Geometry check sheet. Reference: the model listing, model coordinates, mm. A direction names the side the tool comes from. Round coordinates to 2 decimals unless told otherwise and drop trailing zeros. Write each loop counter-clockwise with the first axis right and the second up, starting at its lowest first coordinate (ties: lowest second). Pieces come first, ordered by that corner, then holes. Notation, with made-up numbers: (6, 5.5) -> (15, 5.5) arc R12 cw to (15, 12.5) -> close; hole circle Ø11 at (83.25, -35). An arc over 180 degrees is marked (long way). Use a Markdown table: item, result.
```python
from build123d import *

# Parameters (mm, degrees)
SKETCH1_R           = 1.5
BOSS_EXTRUDE1_DEPTH = 5
FILLET1_R           = 10
CUT_EXTRUDE1_DEPTH  = 1
CUT_EXTRUDE2_DEPTH  = 3.9


with BuildPart() as part:
    # Sketch1 → Boss-Extrude1 (new, symmetric)
    with BuildSketch(Plane.XY):
        with BuildLine():
            Line((4, 60), (4, -60))
            ThreePointArc((4, -60), (0, -64), (-4, -60))
            ThreePointArc((-4, -60), (-12.339895115, 0), (-4, 60))
            ThreePointArc((-4, 60), (0, 64), (4, 60))
        make_face()
        with Locations((0, 60)):
            Circle(SKETCH1_R, mode=Mode.SUBTRACT)
        with Locations((0, 30)):
            Circle(SKETCH1_R, mode=Mode.SUBTRACT)
        with Locations((0, -30)):
            Circle(SKETCH1_R, mode=Mode.SUBTRACT)
        Circle(SKETCH1_R, mode=Mode.SUBTRACT)
        with Locations((0, -60)):
            Circle(SKETCH1_R, mode=Mode.SUBTRACT)
    extrude(amount=BOSS_EXTRUDE1_DEPTH, both=True)

    # Fillet1
    fillet1_edges = [part.edges().sort_by_distance(p)[0] for p in [
        (-4, -60, 0),
        (-4, 60, 0),
    ]]
    fillet(fillet1_edges, radius=FILLET1_R)

    # Sketch2 → Cut-Extrude1 (cut)
    with BuildSketch(Plane.XY.offset(5)):
        with BuildLine():
            ThreePointArc((-3.293906421, -58.816707776), (-0.342834029, -56.516831209), (3, -58.197224362))
            Line((3, -58.197224362), (3, -31.802775638))
            ThreePointArc((3, -31.802775638), (-3.5, -30), (3, -28.197224362))
            Line((3, -28.197224362), (3, -1.802775638))
            ThreePointArc((3, -1.802775638), (-3.5, 0), (3, 1.802775638))
            Line((3, 1.802775638), (3, 28.197224362))
            ThreePointArc((3, 28.197224362), (-3.5, 30), (3, 31.802775638))
            Line((3, 31.802775638), (3, 58.197224362))
            ThreePointArc((3, 58.197224362), (-0.342834029, 56.516831209), (-3.293906421, 58.816707776))
            ThreePointArc((-3.293906421, 58.816707776), (-11.339895115, 0), (-3.293906421, -58.816707776))
        make_face()
    extrude(amount=-CUT_EXTRUDE1_DEPTH, mode=Mode.SUBTRACT)

    # Sketch3 → Cut-Extrude2 (cut, symmetric)
    with BuildSketch(Plane.XY):
        with BuildLine():
            ThreePointArc((-3.293906421, 58.816707776), (-1.64732722, 64.431350021), (0.148659418, 70))
            Line((0.148659418, 70), (-49.851340582, 70))
            Line((-49.851340582, 70), (-49.851340582, -70))
            Line((-49.851340582, -70), (0.148659418, -70))
            ThreePointArc((0.148659418, -70), (-1.64732722, -64.431350021), (-3.293906421, -58.816707776))
            ThreePointArc((-3.293906421, -58.816707776), (-11.339895115, 0), (-3.293906421, 58.816707776))
        make_face()
    extrude(amount=CUT_EXTRUDE2_DEPTH, both=True, mode=Mode.SUBTRACT)


solid = part.part
```
(1) Thickness scan on line 1 (Y direction, x = 0, z = 0.75); line 2 (Y direction, x = -1, z = 0.75); line 3 (Z direction, x = -6.25, y = -48). Record the ranges inside material, lowest first.
A:
| item | result |
|---|---|
| line 1 | y = -64 to -61.5, -58.5 to -31.5, -28.5 to -1.5, 1.5 to 28.5, 31.5 to 58.5, 61.5 to 64 |
| line 2 | y = -63.87 to -61.12, -58.88 to -31.12, -28.88 to -1.12, 1.12 to 28.88, 31.12 to 58.88, 61.12 to 63.87 |
| line 3 | z = -5 to -3.9, 3.9 to 5 |
(2) Section check D-D on y = -11. Record the cut outline in (x, z).
A:
| item | result |
|---|---|
| outline | (-12.06, -5) -> (4, -5) -> (4, 5) -> (3, 5) -> (3, 4) -> (-11.06, 4) -> (-11.06, 5) -> (-12.06, 5) -> (-12.06, 3.9) -> (-11.06, 3.9) -> (-11.06, -3.9) -> (-12.06, -3.9) -> close |
(3) Release check for a two-part mould opening along Y. For faces 1 (the face through (-12.34, -0.84, 4.46)), 2 (the face through (-0.195, -28.513, -0.07)), 3 (the face through (-12, 0, 3.9)) record: +Y half, -Y half, draft (parallel to the pull), parting line (faces both ways), or undercut.
A:
| item | result |
|---|---|
| face 1 | parting line |
| face 2 | undercut |
| face 3 | draft |
(4) Section check C-C on y = 30. Record the cut outline in (x, z), plus the area to 3 significant figures.
A:
| item | result |
|---|---|
| outline | (-10.28, -5) -> (-1.5, -5) -> (-1.5, 5) -> (-3.5, 5) -> (-3.5, 4) -> (-9.28, 4) -> (-9.28, 5) -> (-10.28, 5) -> (-10.28, 3.9) -> (-9.28, 3.9) -> (-9.28, -3.9) -> (-10.28, -3.9) -> close; (1.5, -5) -> (4, -5) -> (4, 5) -> (1.5, 5) -> close |
| area | 99.2 mm2 |
(5) Gauge pin test, flat ends, axial feed: pin 1 Ø2.5 at (x, y) = (0, -30) entering from +Z; pin 2 Ø1.1 at (y, z) = (-44.5, 4.5) entering from -X; pin 3 Ø4.5 at (x, y) = (-3, -9) entering from +Z. Record the tip position at first contact, or that the pin passes through.
A:
| item | result |
|---|---|
| pin 1 | passes through |
| pin 2 | stops at x = -7.91 |
| pin 3 | stops at z = 4 |
(6) Section check A-A on z = 2. Record the cut outline in (x, y).
A:
| item | result |
|---|---|
| outline | (-3.29, -58.82) arc R219 ccw to (-1.93, -63.5) arc R4 ccw to (4, -60) -> (4, 60) arc R4 ccw to (-1.93, 63.5) arc R219 ccw to (-3.29, 58.82) arc R219 ccw to start; hole circle Ø3 at (0, -60); hole circle Ø3 at (0, -30); hole circle Ø3 at (0, 0); hole circle Ø3 at (0, 30); hole circle Ø3 at (0, 60) |
(7) Access from +Z, -Z, +X, -X, +Y, -Y to the whole of each face (thin tool, end or side, straight path). Record for faces 4 (the face through (-4, 1, 4)), 5 (the face through (4, 1, 0)), 6 (the face through (-12, 0, -3.9)).
A:
| item | result |
|---|---|
| face 4 | +Z |
| face 5 | +Z, -Z, +X, +Y, -Y |
| face 6 | -X |
(8) Section check B-B on y = 8. Record the cut outline in (x, z).
A:
| item | result |
|---|---|
| outline | (-12.19, -5) -> (4, -5) -> (4, 5) -> (3, 5) -> (3, 4) -> (-11.19, 4) -> (-11.19, 5) -> (-12.19, 5) -> (-12.19, 3.9) -> (-11.19, 3.9) -> (-11.19, -3.9) -> (-12.19, -3.9) -> close |
